Geometry: final body of the model. Coordinates: model frame, mm. Face numbers are marked on the shaded views. Round coordinates to 2 decimals unless told otherwise and drop trailing zeros. Loops run counter-clockwise (first coordinate to the right, second up) from the corner with the lowest first, then second, coordinate; pieces in that order, holes last. Notation, with made-up numbers: (-35, -22.5) - (0, -22.5) arc R11 ccw to (0, -2.5) - close; hole circle Ø5 at (-12.75, 22.5). An arc over 180 degrees is marked (long way). Return JSON: item names as keys, results as strings. Group by question number.
1. Material intervals for probe 1 along X at (y, z) = (288.5, 1); probe 2 along X at (y, z) = (118.5, 15.5); probe 3 along Y at (x, z) = (-112.5, 3), sorted ascending.
2. Draft query along X for the marked faces 1 and 2. Return one class per face: +X half, -X half, draft (parallel to the pull), parting line (faces both ways), or undercut.
3. Section C-C on x = 92.5. Return loops of the section in (y, z), and give its area (3 significant figures).
4. Section B-B on z = 7.5. Return loops of the section in (x, y).
5. Section A-A on y = 119. Return loops of the section in (x, z), and give its area (3 significant figures).
6. Section D-D on y = -86. Return loops of the section in (x, z).
from build123d import *

# Parameters (mm, degrees)
F0_W     = 1200
F0_H     = 800
F1_DEPTH = 21
F2_W     = 250
F2_H     = 500
F3_DEPTH = 15
F4_R     = 8
F5_R     = 8
F6_R     = 8
F7_R     = 8
F8_W     = 3
F8_H     = 200
F9_DEPTH = 25


with BuildPart() as f1:
    # F0 (on Top) → F1 (new body)
    with BuildSketch(Plane.XY):
        with Locations((-0.654887, 101.971073)):
            Rectangle(F0_W, F0_H)
    extrude(amount=F1_DEPTH)

    # F2 (on face) → F3 (cut)
    with BuildSketch(Plane(origin=(0, 0, 0), x_dir=(1, 0, 0), z_dir=(0, 0, -1))):
        with Locations((-0.654887, -51.971073)):
            Rectangle(F2_W, F2_H)
    extrude(amount=-F3_DEPTH, mode=Mode.SUBTRACT)

    # F4
    f4_edges = [f1.edges().sort_by_distance(p)[0] for p in [
        (-125.654887, -198.028927, 7.5),
    ]]
    fillet(f4_edges, radius=F4_R)

    # F5
    f5_edges = [f1.edges().sort_by_distance(p)[0] for p in [
        (124.345113, 301.971073, 7.5),
    ]]
    fillet(f5_edges, radius=F5_R)

    # F6
    f6_edges = [f1.edges().sort_by_distance(p)[0] for p in [
        (124.345113, -198.028927, 7.5),
    ]]
    fillet(f6_edges, radius=F6_R)

    # F7
    f7_edges = [f1.edges().sort_by_distance(p)[0] for p in [
        (-125.654887, 301.971073, 7.5),
    ]]
    fillet(f7_edges, radius=F7_R)

    # F8 (on face) → F9 (cut)
    with BuildSketch(Plane(origin=(0, 0, 15), x_dir=(1, 0, 0), z_dir=(0, 0, -1))):
        with Locations((122.845113, -51.971073)):
            Rectangle(F8_W, F8_H)
    extrude(amount=-F9_DEPTH, mode=Mode.SUBTRACT)


solid = f1.part
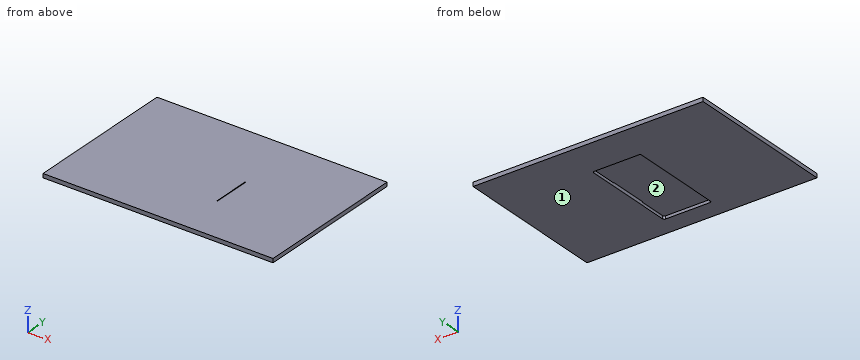
Taken from the geometry:
{
 "1": {"probe 1": "-600.65 to -125.65, 124.35 to 599.35", "probe 2": "-600.65 to 121.35, 124.35 to 599.35", "probe 3": "-298.03 to -198.03, 301.97 to 501.97"},
 "2": {"face 1": "draft", "face 2": "undercut"},
 "3": {"outline": "(-298.03, 0) - (-198.03, 0) - (-198.03, 15) - (301.97, 15) - (301.97, 0) - (501.97, 0) - (501.97, 21) - (-298.03, 21) - close", "area": "9,300 mm2"},
 "4": {"outline": "(-600.65, -298.03) - (599.35, -298.03) - (599.35, 501.97) - (-600.65, 501.97) - close; hole (-125.65, -190.03) arc R8 ccw to (-117.65, -198.03) - (116.35, -198.03) arc R8 ccw to (124.35, -190.03) - (124.35, 293.97) arc R8 ccw to (116.35, 301.97) - (-117.65, 301.97) arc R8 ccw to (-125.65, 293.97) - close"},
 "5": {"outline": "(-600.65, 0) - (-125.65, 0) - (-125.65, 15) - (121.35, 15) - (121.35, 21) - (-600.65, 21) - close; (124.35, 0) - (599.35, 0) - (599.35, 21) - (124.35, 21) - close", "area": "21,400 mm2"},
 "6": {"outline": "(-600.65, 0) - (-125.65, 0) - (-125.65, 15) - (124.35, 15) - (124.35, 0) - (599.35, 0) - (599.35, 21) - (-600.65, 21) - close"}
}
